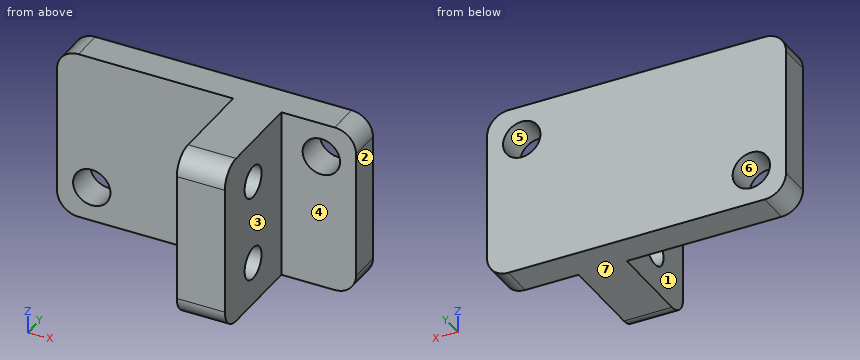
from build123d import *

# Parameters (mm, degrees)
F0_R     = 1.75
F1_DEPTH = 1.5
F4_DEPTH = 3
F5_DEPTH = 1.5
F6_R     = 1.5
F7_DEPTH = 21.001


with BuildPart() as f1:
    # F0 (on Front) → F1 (new body, symmetric)
    with BuildSketch(Plane.XZ):
        with BuildLine():
            ThreePointArc((14, 6), (13.4142135624, 7.4142135624), (12, 8))
            Line((12, 8), (-12, 8))
            ThreePointArc((-12, 8), (-13.4142135624, 7.4142135624), (-14, 6))
            Line((-14, 6), (-14, -6))
            ThreePointArc((-14, -6), (-13.4142135624, -7.4142135624), (-12, -8))
            Line((-12, -8), (12, -8))
            ThreePointArc((12, -8), (13.4142135624, -7.4142135624), (14, -6))
            Line((14, -6), (14, 6))
        make_face()
        with Locations((-10.75, -4.75)):
            Circle(F0_R, mode=Mode.SUBTRACT)
        with Locations((10.75, 4.75)):
            Circle(F0_R, mode=Mode.SUBTRACT)
    extrude(amount=F1_DEPTH, both=True)

    # F3 (on offset) → F4 (join)
    with BuildSketch(Plane.YZ.offset(4)):
        with BuildLine():
            Line((-9.5, -8), (-1.5, -8))
            Line((-1.5, -8), (-1.5, 8))
            Line((-1.5, 8), (-9.5, 8))
            ThreePointArc((-9.5, 8), (-10.9142135624, 7.4142135624), (-11.5, 6))
            Line((-11.5, 6), (-11.5, -6))
            ThreePointArc((-11.5, -6), (-10.9142135624, -7.4142135624), (-9.5, -8))
        make_face()
    extrude(amount=F4_DEPTH)

    # F3 (on offset) → F5 (join, symmetric)
    with BuildSketch(Plane.YZ.offset(4)):
        with BuildLine():
            Line((-9.5, -8), (-1.5, -8))
            Line((-1.5, -8), (-1.5, 8))
            Line((-1.5, 8), (-9.5, 8))
            ThreePointArc((-9.5, 8), (-10.9142135624, 7.4142135624), (-11.5, 6))
            Line((-11.5, 6), (-11.5, -6))
            ThreePointArc((-11.5, -6), (-10.9142135624, -7.4142135624), (-9.5, -8))
        make_face()
    extrude(amount=F5_DEPTH, both=True)

    # F6 (on face) → F7 (cut, through all)
    with BuildSketch(Plane.YZ.offset(7)):
        with Locations((-6.5, 4)):
            Circle(F6_R)
        with Locations((-6.5, -4)):
            Circle(F6_R)
    extrude(amount=-F7_DEPTH, mode=Mode.SUBTRACT)


solid = f1.part
Source: CAD feature listing. Evaluate the final solid. Frame: model axes, mm. Face numbers are marked on the shaded views. A direction names the side the tool comes from. Round coordinates to 2 decimals unless told otherwise and drop trailing zeros. Loops run counter-clockwise (first coordinate to the right, second up) from the corner with the lowest first, then second, coordinate; pieces in that order, holes last. Notation, with made-up numbers: (42, 80.5) -> (95, 80.5) arc R22 ccw to (95, 103.5) -> close; hole circle Ø7 at (38, 14.25). An arc over 180 degrees is marked (long way). Answer as a JSON object with one key per item and string values. Group by question number.
Q1. Section query D-D (y = -9). Output: boundary loops of the cut face in (x, z), plus the area to 3 significant figures.
Q2. Contact query for flat-ended pins moving along their axis: P1, Ø8, axis at x = -7, z = 2.5, coming from the -Y side; P2, Ø6, axis at y = -6, z = -3, coming from the -X side; P3, Ø3, axis at x = -10.75, z = -4.75, coming from the -Y side; P4, Ø4, axis at y = -6.5, z = 4, coming from the +X side. Output: stop coordinate, or through.
Q3. Ray query, line 1 (Z direction, x = 3.7, y = -6.5); line 2 (Z direction, x = 10.75, y = 0.8); line 3 (X direction, y = -3.25, z = 5.5). Return the intervals inside material, ascending. Write a range as from..to.
Q4. Section query B-B (z = -4). Output: boundary loops of the cut face in (x, y), plus the area to 3 significant figures.
Q5. Mould query, pull axis Z, two halves, no side actions, for the marked faces 4, 5, 6 and 7. Classes: pulls with the +Z half, pulls with the -Z half, needs draft (parallel to the pull), parting line crosses it, or undercut.
Q6. Access query for the marked faces 1, 2 and 3. Directions: +Z, -Z, +X, -X, +Y, -Y. A direction counts if a zero-diameter tool reaches every point of the face in a straight line with its end or side. Return the directions, or none.
Q7. Section query A-A (x = 10.75). Output: boundary loops of the cut face in (y, z).
Q8. Section query C-C (y = -0.25). Output: boundary loops of the cut face in (x, z).
Completed:
{
 "1": {"outline": "(2.5, -8) -> (7, -8) -> (7, 8) -> (2.5, 8) -> close", "area": "72.0 mm²"},
 "2": {"P1": "y = -1.5", "P2": "x = 2.5", "P3": "through", "P4": "x = 7"},
 "3": {"line 1": "-8..-5.5, -2.5..2.5, 5.5..8", "line 2": "-8..3, 6.5..8", "line 3": "2.5..7"},
 "4": {"outline": "(-14, -1.5) -> (-12.33, -1.5) -> (-12.33, 1.5) -> (-14, 1.5) -> close; (-9.17, -1.5) -> (2.5, -1.5) -> (2.5, -5) -> (7, -5) -> (7, -1.5) -> (14, -1.5) -> (14, 1.5) -> (-9.17, 1.5) -> close; (2.5, -11.5) -> (7, -11.5) -> (7, -8) -> (2.5, -8) -> close", "area": "106 mm²"},
 "5": {"face 4": "needs draft", "face 5": "undercut", "face 6": "undercut", "face 7": "pulls with the -Z half"},
 "6": {"face 1": "+Z, -Z, -X, -Y", "face 2": "+Z, -Z, +X, +Y, -Y", "face 3": "+Z, -Z, +X, -Y"},
 "7": {"outline": "(-1.5, -8) -> (1.5, -8) -> (1.5, 3) -> (-1.5, 3) -> close; (-1.5, 6.5) -> (1.5, 6.5) -> (1.5, 8) -> (-1.5, 8) -> close"},
 "8": {"outline": "(-14, -6) arc R2 ccw to (-12, -8) -> (12, -8) arc R2 ccw to (14, -6) -> (14, 6) arc R2 ccw to (12, 8) -> (-12, 8) arc R2 ccw to (-14, 6) -> close; hole circle Ø3.5 at (-10.75, -4.75); hole circle Ø3.5 at (10.75, 4.75)"}
}
